```python
from build123d import *

# Parameters (mm, degrees)
CROQUIS1_R              = 1.75
CROQUIS1_R_2            = 3.5
CROQUIS1_R_3            = 2
CROQUIS1_R_4            = 1.5
SALIENTE_EXTRUIR1_DEPTH = 3


with BuildPart() as part:
    # Croquis1 → Saliente-Extruir1 (new body)
    with BuildSketch(Plane(origin=(0, 0, 0), x_dir=(0, 0, -1), z_dir=(1, 0, 0))):
        with BuildLine():
            ThreePointArc((-12.479760771, -8.321993217), (10.178991806, -11.017627957), (9.281950646, 11.783267467))
            add(Edge.make_bspline(
                [(-153.589400871, 9.333606023), (-52.027464553, 57.017454048), (-3.028685523, 21.666117386), (9.281950646, 11.783267467)],
                knots=[0, 0, 0, 0, 1, 1, 1, 1], degree=3))
            ThreePointArc((-153.589400871, 9.333606023), (-158.998047864, -4.362927301), (-144.894564169, -8.598518767))
            add(Edge.make_bspline(
                [(-144.894564169, -8.598518767), (-94.399563679, 13.089335746), (-29.021790265, 9.608207487), (-12.479760771, -8.321993217)],
                knots=[0, 0, 0, 0, 1, 1, 1, 1], degree=3))
        make_face()
        with Locations((-150, 0)):
            Circle(CROQUIS1_R, mode=Mode.SUBTRACT)
        Circle(CROQUIS1_R_2, mode=Mode.SUBTRACT)
        with Locations((-113, 13.11718)):
            Circle(CROQUIS1_R_3, mode=Mode.SUBTRACT)
        with Locations((-30, 15.614781046)):
            Circle(CROQUIS1_R_3, mode=Mode.SUBTRACT)
        with Locations((-7.5, 0)):
            Circle(CROQUIS1_R_4, mode=Mode.SUBTRACT)
        with Locations((0, -7.5)):
            Circle(CROQUIS1_R_4, mode=Mode.SUBTRACT)
        with Locations((0, 7.5)):
            Circle(CROQUIS1_R_4, mode=Mode.SUBTRACT)
        with Locations((7.5, 0)):
            Circle(CROQUIS1_R_4, mode=Mode.SUBTRACT)
    extrude(amount=SALIENTE_EXTRUIR1_DEPTH)


solid = part.part
```
Geometry: final body of the model. Coordinates: model frame, mm. Give positions to 0.01 mm unless a question says otherwise; leave off trailing zeros. Write each question's results on one line, items separated by ' | '. Start each with the question number.
1) Draft query along Z for faces 1 (the cylindrical face through (1, -9, 0)), 2 (the flat face through (0, 13, 66)). Return one class per face: pulls with the +Z half, pulls with the -Z half, needs draft (parallel to the pull), parting line crosses it, or undercut.
2) First-contact query: pin 1 (5 mm diameter, centred on y = 7.5, z = 0, fed in from -X). Flat tip, straight axial feed; report the tip coordinate or a pass-through.
3) Section A-A (y = 0). Count the separate pieces of the cut face and the enclosed holes in it, then the cut area to 3 significant figures.
4) Line query: line 1 (Y direction, x = 1.75, z = 0); line 2 (Y direction, x = 1.1, z = 151); line 3 (Y direction, x = 1.5, z = 23). Output: solid intervals per line, ascending. Write a range as from..to.
Calculated:
1) face 1: undercut | face 2: needs draft
2) pin 1: x = 0
3) separate pieces: 6 | enclosed holes: 0 | area: 195 mm2
4) line 1: -15..-9, -6..-3.5, 3.5..6, 9..18.34 | line 2: -9.95..-1.44, 1.44..10.54 | line 3: -1.27..28.59
